Work out the finished part from the listing and answer in its coordinate system (mm). Coordinates: 2 decimals unless noted, no trailing zeros. Write each question's results on one line, items separated by ' | '. Start each with the question number.
Item 1: Consider probe 1 along Z at (x, y) = (10, -0.35); probe 2 along Z at (x, y) = (9.5, -0.2); probe 3 along Z at (x, y) = (12, -0.25). Determine where each line is inside the solid, lowest interval first. Write a range as [from, to].
Item 2: This flat-tipped pin is pushed along its axis until it touches: pin 1 Ø5.5 at (x, z) = (10, 600) entering from +Y. Where does it stop, or does it pass through?
Item 3: For a pull along Y with two mould halves and no side action, classify faces 1 (the face through (10, 0, 309)), 2 (the face through (10, -1, 309)) as +Y half, -Y half, draft (parallel to the pull), parting line (faces both ways), or undercut.
from build123d import *

# Parameters (mm, degrees)
F0_R     = 3
F0_R_2   = 1.6
F1_DEPTH = 1


with BuildPart() as f1:
    # F0 (on Front) → F1 (new body)
    with BuildSketch(Plane.XZ):
        with BuildLine():
            ThreePointArc((0, 5), (1.464466, 1.464466), (5, 0))
            Line((5, 0), (15, 0))
            ThreePointArc((15, 0), (18.535534, 1.464466), (20, 5))
            Line((20, 5), (20, 605))
            ThreePointArc((20, 605), (18.535534, 608.535534), (15, 610))
            Line((15, 610), (5, 610))
            ThreePointArc((5, 610), (1.464466, 608.535534), (0, 605))
            Line((0, 605), (0, 5))
        make_face()
        with Locations((10, 10)):
            Circle(F0_R, mode=Mode.SUBTRACT)
        with Locations((10, 405.2)):
            Circle(F0_R_2, mode=Mode.SUBTRACT)
        with Locations((10, 562.68)):
            Circle(F0_R_2, mode=Mode.SUBTRACT)
        with Locations((10, 600)):
            Circle(F0_R, mode=Mode.SUBTRACT)
    extrude(amount=F1_DEPTH)


solid = f1.part
Answer key:
1) probe 1: z = [0, 7], [13, 403.6], [406.8, 561.08], [564.28, 597], [603, 610] | probe 2: z = [0, 7.04], [12.96, 403.68], [406.72, 561.16], [564.2, 597.04], [602.96, 610] | probe 3: z = [0, 7.76], [12.24, 597.76], [602.24, 610]
2) pin 1: passes through
3) face 1: +Y half | face 2: -Y half
